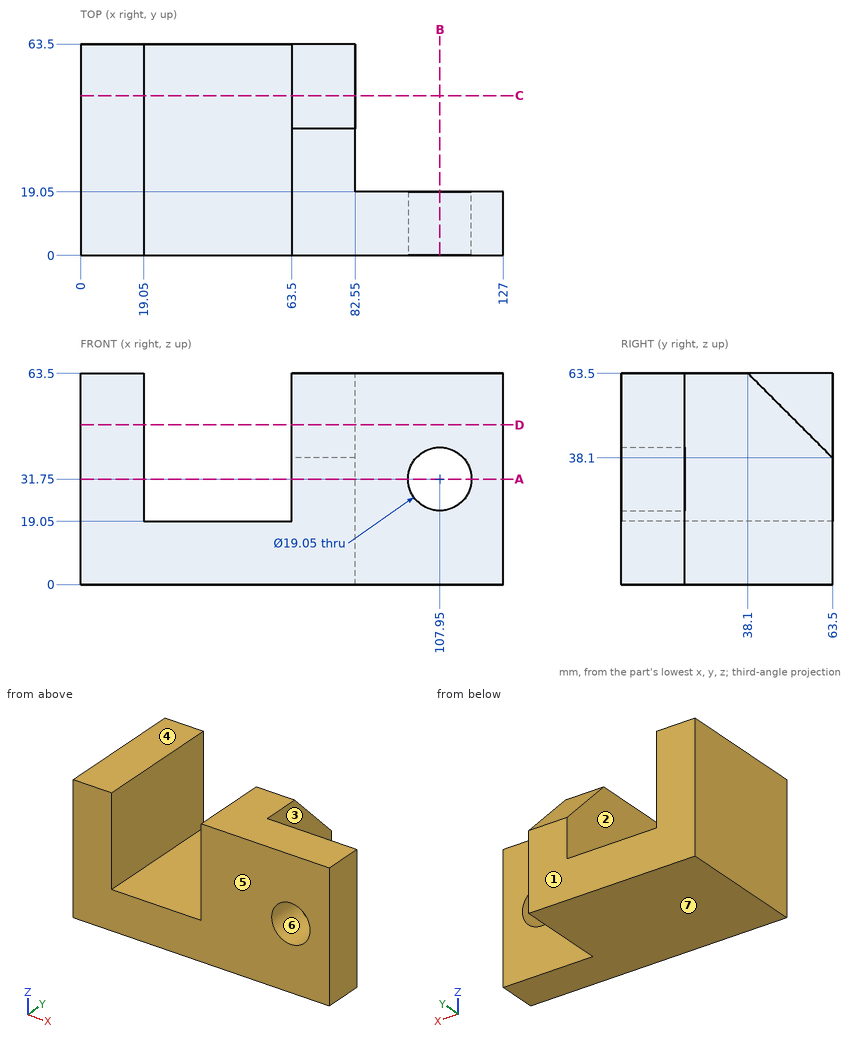
Here's the drawing with two shaded views (mm, measured from the low corner). I have some questions. A direction names the side the tool comes from. Coordinates: 2 decimals unless noted, no trailing zeros. Write each loop counter-clockwise with the first axis right and the second up, starting at its lowest first coordinate (ties: lowest second). Pieces come first, ordered by that corner, then holes. Notation, with made-up numbers: (54, 18.25) -> (67, 18.25) arc R16 ccw to (67, 33.25) -> close; hole circle Ø3 at (-5, -12). An arc over 180 degrees is marked (long way). Use a Markdown table: item, result. Add a question column.
(1) I'm going to push flat-ended pins straight in: P1, Ø5, axis at x = 65.5, y = 14, coming from the -Z side; P2, Ø13.5, axis at x = 97, z = 37, coming from the +Y side. Where does each tip first touch, or does it pass through?
(2) If we section it at B-B, the plane x = 107.95: Write out the boundary of the cut face in (y, z) (3 decimals), and give its area (3 significant figures).
(3) For the marked faces 1, 2 and 3, which set-ups out of +Z, -Z, +X, -X, +Y, -Y let a thin tool reach every point of the face, with its end or its side?
(4) If we section it at A-A, the plane z = 31.75: Write out the boundary of the cut face in (x, y) (3 decimals).
(5) We'd pull the mould along Z, two halves only. Please class the marked faces 4, 5, 6 and 7: +Z half, -Z half, draft (parallel to the pull), parting line (faces both ways), or undercut.
(6) If we section it at C-C, the plane y = 48: Write out the boundary of the cut face in (x, z), and give its area (3 significant figures).
(7) If we section it at D-D, the plane z = 48: Write out the boundary of the cut face in (x, y), and give its area (3 significant figures).
(8) Please list where these lines run through material, in increasing order: line 1 (X direction, y = 13, z = 31); line 2 (X direction, y = 35, z = 35); line 3 (Z direction, x = 107.95, y = 8.5) (3 decimals).
Outcome:
| question | item | result |
|---|---|---|
| 1 | P1 | stops at z = 0 |
| 1 | P2 | stops at y = 19.05 |
| 2 | outline | (0, 0) -> (19.05, 0) -> (19.05, 22.225) -> (0, 22.225) -> close; (0, 41.275) -> (19.05, 41.275) -> (19.05, 63.5) -> (0, 63.5) -> close |
| 2 | area | 847 mm^2 |
| 3 | face 1 | +Z, -Z, +X, -X, +Y |
| 3 | face 2 | +Z, +Y, -Y |
| 3 | face 3 | +Z, -Z, +X, +Y |
| 4 | outline | (0, 0) -> (19.05, 0) -> (19.05, 63.5) -> (0, 63.5) -> close; (63.5, 0) -> (98.425, 0) -> (98.425, 19.05) -> (82.55, 19.05) -> (82.55, 63.5) -> (63.5, 63.5) -> close; (117.475, 0) -> (127, 0) -> (127, 19.05) -> (117.475, 19.05) -> close |
| 5 | face 4 | +Z half |
| 5 | face 5 | draft |
| 5 | face 6 | undercut |
| 5 | face 7 | -Z half |
| 6 | outline | (0, 0) -> (82.55, 0) -> (82.55, 53.6) -> (63.5, 53.6) -> (63.5, 19.05) -> (19.05, 19.05) -> (19.05, 63.5) -> (0, 63.5) -> close |
| 6 | area | 3,080 mm^2 |
| 7 | outline | (0, 0) -> (19.05, 0) -> (19.05, 63.5) -> (0, 63.5) -> close; (63.5, 0) -> (127, 0) -> (127, 19.05) -> (82.55, 19.05) -> (82.55, 53.6) -> (63.5, 53.6) -> close |
| 7 | area | 3,080 mm^2 |
| 8 | line 1 | x = 0 to 19.05, 63.5 to 98.45, 117.45 to 127 |
| 8 | line 2 | x = 0 to 19.05, 63.5 to 82.55 |
| 8 | line 3 | z = 0 to 22.225, 41.275 to 63.5 |
